from build123d import *
from build123d.topology import SkipClean

# Parameters (mm, degrees)
BOSS_EXTRUDE1_DEPTH     = 50
BOSS_EXTRUDE2_START     = 9
BOSS_EXTRUDE2_DEPTH     = 9
BOSS_EXTRUDE3_START     = 9
BOSS_EXTRUDE3_DEPTH     = 9
BOSS_EXTRUDE4_DEPTH     = 70
CUT_EXTRUDE2_DEPTH      = 165.74298164110058
CUT_EXTRUDE2_DEPTH_BACK = 165.74298164110058
SKETCH10_W              = 30.000000000000007
SKETCH10_H              = 30
SKETCH10_W_2            = 30.00000000000001
SKETCH10_H_2            = 29.999999999999996
BOSS_EXTRUDE7_DEPTH     = 90
BOSS_EXTRUDE8_DEPTH     = 235
SKETCH12_W              = 24.999999999999993
SKETCH12_H              = 40.90326072663956
SKETCH12_H_2            = 38.73852460954424
SKETCH12_W_2            = 25.000000000000007
SKETCH12_H_3            = 39.91957718910348
CUT_EXTRUDE3_DEPTH      = 235
SKETCH13_R              = 7.499999999999999
CUT_EXTRUDE4_DEPTH      = 235
FILLET1_R               = 10


with BuildPart() as part:
    # Sketch1 → Boss-Extrude1 (new body)
    with BuildSketch(Plane(origin=(0, 0, 0), x_dir=(0, 0, -1), z_dir=(1, 0, 0))):
        with BuildLine():
            Line((-130.5, 0), (130.5, 0))
            ThreePointArc((130.5, 0), (137.57106781186548, -2.9289321881345245), (140.5, -9.999999999999998))
            Line((140.5, -9.999999999999998), (140.5, -69.99999999999999))
            Line((140.5, -69.99999999999999), (122.5, -70))
            ThreePointArc((122.5, -70), (97.5, -45), (72.50000000000001, -70))
            Line((72.50000000000001, -70), (57.5, -70))
            ThreePointArc((57.5, -70), (32.5, -45), (7.5, -70))
            Line((7.5, -70), (-7.5, -70))
            ThreePointArc((-7.5, -70), (-32.5, -45), (-57.5, -70))
            Line((-57.5, -70), (-72.50000000000001, -70))
            ThreePointArc((-72.50000000000001, -70), (-97.5, -45), (-122.5, -70))
            Line((-122.5, -70), (-140.5, -69.99999999999999))
            Line((-140.5, -69.99999999999999), (-140.5, -9.999999999999998))
            ThreePointArc((-140.5, -9.999999999999998), (-137.57106781186548, -2.9289321881345245), (-130.5, 0))
        make_face()
    extrude(amount=BOSS_EXTRUDE1_DEPTH)

    # Sketch2 → Boss-Extrude2 (add)
    with BuildSketch(Plane.ZY.offset(BOSS_EXTRUDE2_START)):
        with BuildLine():
            Line((0, 0), (130.5, 0))
            ThreePointArc((130.5, 0), (137.57106781186548, -2.9289321881345236), (140.5, -9.999999999999998))
            Line((140.5, -9.999999999999998), (140.5, -69.99999999999999))
            Line((140.5, -69.99999999999999), (135.5, -69.99999999999999))
            Line((135.5, -69.99999999999999), (135.5, -15))
            ThreePointArc((135.5, -15), (132.57106781186548, -7.928932188134525), (125.5, -5.000000000000002))
            Line((125.5, -5.000000000000002), (0, -5.000000000000017))
            Line((0, -5.000000000000017), (0, 0))
        make_face()
    extrude(amount=-BOSS_EXTRUDE2_DEPTH)

    # Sketch3 → Boss-Extrude3 (add)
    with BuildSketch(Plane.ZY.offset(BOSS_EXTRUDE3_START)):
        with BuildLine():
            Line((0, 0), (0, -5.000000000000017))
            Line((0, -5.000000000000017), (-125.5, -5.000000000000032))
            ThreePointArc((-125.5, -5.000000000000032), (-132.57106781186548, -7.9289321881345565), (-135.5, -15.000000000000034))
            Line((-135.5, -15.000000000000034), (-135.5, -69.99999999999999))
            Line((-135.5, -69.99999999999999), (-140.5, -69.99999999999999))
            Line((-140.5, -69.99999999999999), (-140.5, -10.00000000000007))
            ThreePointArc((-140.5, -10.00000000000007), (-137.5710678118655, -2.9289321881345742), (-130.50000000000003, 5.2e-15))
            Line((-130.50000000000003, 5.2e-15), (0, 0))
        make_face()
    extrude(amount=-BOSS_EXTRUDE3_DEPTH)

    # Sketch6 → Boss-Extrude4 (add)
    with BuildSketch(Plane(origin=(0, 0, 0), x_dir=(1, 0, 0), z_dir=(0, 1, 0))):
        Polygon((50, -140.5), (50, 140.5), (43, 140.5), (43.000000000000036, -140.5), align=None)
    extrude(amount=-BOSS_EXTRUDE4_DEPTH)

    # Sketch9 → Cut-Extrude2 (cut, two sides: drawn at the far end of the back side and taken through both)
    with BuildSketch(Plane(origin=(0, 0, 0), x_dir=(1, 0, 0), z_dir=(0, 1, 0)).offset(-CUT_EXTRUDE2_DEPTH_BACK)):
        Polygon((40.000000000000675, 47.5), (40.00000000000068, 17.49999999999999), (10.000000000000675, 17.49999999999999), (10.000000000000671, 47.499999999999986), align=None)
        Polygon((39.99999999999999, 112.5), (9.999999999999995, 112.49999999999999), (9.999999999999998, 82.49999999999999), (40, 82.49999999999999), align=None)
        Polygon((40.00000000000135, -17.5), (40.00000000000136, -47.500000000000014), (10.000000000001352, -47.500000000000014), (10.000000000001348, -17.500000000000014), align=None)
        Polygon((40.000000000002025, -82.5), (40.00000000000203, -112.50000000000001), (10.00000000000203, -112.50000000000001), (10.000000000002027, -82.50000000000001), align=None)
    extrude(amount=CUT_EXTRUDE2_DEPTH + CUT_EXTRUDE2_DEPTH_BACK, mode=Mode.SUBTRACT)

    # Sketch10 → Boss-Extrude7 (add)
    # profile 1 of 4: a face of its own
    with BuildSketch(Plane(origin=(0, 0, 0), x_dir=(1, 0, 0), z_dir=(0, 1, 0))):
        Polygon((4.99999999999999, 117.5), (44.99999999999999, 117.5), (45, 77.49999999999999), (4.999999999999995, 77.49999999999999), align=None)
        with Locations((24.999999999999996, 97.49999999999999)):
            Rectangle(SKETCH10_W, SKETCH10_H, mode=Mode.SUBTRACT)
    # profile 2 of 4: a face of its own
    with BuildSketch(Plane(origin=(0, 0, 0), x_dir=(1, 0, 0), z_dir=(0, 1, 0))):
        Polygon((5.000000000000667, 52.49999999999999), (5.0000000000006715, 12.499999999999984), (45.000000000000675, 12.499999999999984), (45.00000000000067, 52.49999999999999), align=None)
        with Locations((25.000000000000675, 32.499999999999986)):
            Rectangle(SKETCH10_W_2, SKETCH10_H_2, mode=Mode.SUBTRACT)
    # profile 3 of 4: a face of its own
    with BuildSketch(Plane(origin=(0, 0, 0), x_dir=(1, 0, 0), z_dir=(0, 1, 0))):
        Polygon((5.000000000001345, -12.50000000000001), (5.000000000001349, -52.50000000000002), (45.00000000000135, -52.50000000000002), (45.00000000000134, -12.50000000000001), align=None)
        with Locations((25.000000000001354, -32.500000000000014)):
            Rectangle(SKETCH10_W, SKETCH10_H, mode=Mode.SUBTRACT)
    # profile 4 of 4: a face of its own
    with BuildSketch(Plane(origin=(0, 0, 0), x_dir=(1, 0, 0), z_dir=(0, 1, 0))):
        Polygon((5.0000000000020215, -77.50000000000001), (5.000000000002025, -117.50000000000001), (45.00000000000203, -117.50000000000001), (45.000000000002025, -77.50000000000001), align=None)
        with Locations((25.00000000000203, -97.50000000000001)):
            Rectangle(SKETCH10_W, SKETCH10_H, mode=Mode.SUBTRACT)
    extrude(amount=BOSS_EXTRUDE7_DEPTH)

    # Sketch11 → Boss-Extrude8 (add)
    with BuildSketch(Plane.XY.offset(117.50000000000001)):
        with BuildLine():
            Line((45.00000000000203, 59.449874371066194), (45.00000000000203, 56.93303437365923))
            ThreePointArc((45.00000000000203, 56.93303437365923), (53.50000000000204, 49.499999999999986), (45.00000000000203, 42.06696562634074))
            Line((45.00000000000203, 42.06696562634074), (45.00000000000203, 39.55012562893379))
            ThreePointArc((45.00000000000203, 39.5501256289338), (56.000000000002046, 49.5), (45.00000000000203, 59.4498743710662))
        make_face()
    extrude(amount=-BOSS_EXTRUDE8_DEPTH)

    # Sketch12 → Cut-Extrude3 (cut)
    with BuildSketch(Plane(origin=(0, 0, 0), x_dir=(0, 0, -1), z_dir=(1, 0, 0))):
        with Locations((-65.00000000000001, 54.273306822213314)):
            Rectangle(SKETCH12_W, SKETCH12_H)
        with Locations((-1.421e-14, 51.301254636370814)):
            Rectangle(SKETCH12_W, SKETCH12_H_2)
        with Locations((65, 47.16757060791335)):
            Rectangle(SKETCH12_W_2, SKETCH12_H_3)
    extrude(amount=CUT_EXTRUDE3_DEPTH, mode=Mode.SUBTRACT)

    # Sketch13 → Cut-Extrude4 (cut)
    with SkipClean():  # the faces are left unmerged after this step: merging them gives an invalid solid
        with BuildSketch(Plane.XY.offset(117.50000000000001)):
            with Locations((46.000000000002046, 49.499999999999986)):
                Circle(SKETCH13_R)
        extrude(amount=-CUT_EXTRUDE4_DEPTH, mode=Mode.SUBTRACT)

    # Fillet1
    fillet1_edges = [part.edges().sort_by_distance(p)[0] for p in [
        (46.500000000000014, 0, 140.5),
        (46.5, 0, -140.5),
    ]]
    fillet(fillet1_edges, radius=FILLET1_R)


solid = part.part
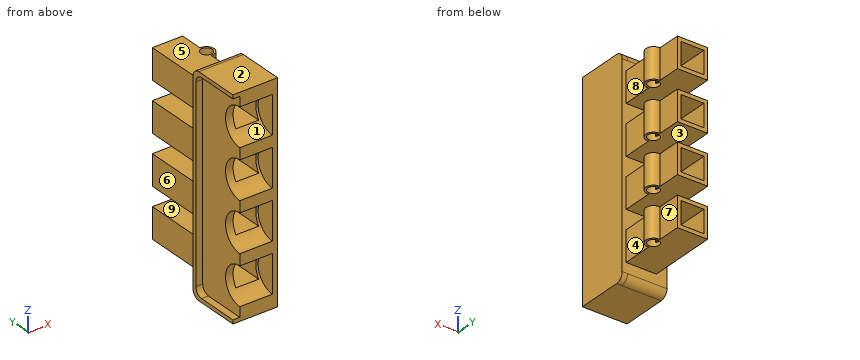
Input: part model. Units: mm. Frame: model coordinates. Face numbers are marked on the shaded views. A direction names the side the tool comes from. Round coordinates to 2 decimals unless told otherwise and drop trailing zeros. Loops run counter-clockwise (first coordinate to the right, second up) from the corner with the lowest first, then second, coordinate; pieces in that order, holes last. Notation, with made-up numbers: M 8,70.5 L 33,70.5 A24 ccw 33,88.5 Z; hole C -18,45.25 d2. An arc over 180 degrees is marked long. Answer as CSV lines item,"result". Start each with the question number.
(1) Reachability of the marked faces 5, 6, 7, 8 and 9 from +Z, -Z, +X, -X, +Y, -Y: full face, straight path, thin tool, end or side. Return the list, or none.
(2) Section C-C, the plane y = -41.5. Output: boundary loops of the cut face in (x, z).
(3) Section B-B, the plane z = -32.5. Output: boundary loops of the cut face in (x, y), plus the area to 3 significant figures.
(4) Section A-A, the plane y = 62.5. State how many separate pieces and enclosed holes the cut face has, plus the area to 3 significant figures.
(5) Draft query along Z for the marked faces 1, 2, 3 and 4. Return one class per face: released by +Z, released by -Z, zero draft, split by the parting line, or undercut.
(6) Line query: line 1 (Z direction, x = 35.5, y = -24); line 2 (Z direction, x = 41.5, y = 26); line 3 (Y direction, x = 46, z = -32). Output: solid intervals per line, ascending. Write a range as [from, to].
(7) First-contact query: pin 1 (8 mm diameter, centred on x = 23, y = 33, fed in from +Z); pin 2 (8 mm diameter, centred on y = 10, z = 102, fed in from +X); pin 3 (10 mm diameter, centred on x = 44.5, y = 54.5, fed in from -Z). Flat tips, straight axial feed; report the tip coordinate or a pass-through.
Values found:
1,face 5,"+Z, +X, -X, +Y"
1,face 6,"+Z, -Z, -X, +Y"
1,face 7,"+Z, -Z, +X, +Y"
1,face 8,"+Z, -Z, +X"
1,face 9,"+X, -X, +Y"
2,outline,"M -9,-140.5 L 50,-140.5 L 50,140.5 L -9,140.5 L -9,135.5 L 0,135.5 L 0,-135.5 L -9,-135.5 Z; hole M 10,-112.5 L 40,-112.5 L 40,-82.5 L 10,-82.5 Z; hole M 10,-47.5 L 40,-47.5 L 40,-17.5 L 10,-17.5 Z; hole M 10,17.5 L 40,17.5 L 40,47.5 L 10,47.5 Z; hole M 10,82.5 L 40,82.5 L 40,112.5 L 10,112.5 Z"
3,outline,"M -9,-5 L 0,-5 L 0,-45 L 10,-45 L 10,90 L 5,90 L 5,0 L -9,0 Z; M 40,-45 L 43,-45 L 43,-70 L 50,-70 L 50,0 L 45,0 L 45,39.55 A10 ccw long 45,59.45 L 45,90 L 40,90 L 40,54 A7.5 cw long 40,45 Z"
3,area,"2,030 mm²"
4,separate pieces,"4"
4,enclosed holes,"4"
4,area,"2,800 mm²"
5,face 1,"undercut"
5,face 2,"released by +Z"
5,face 3,"undercut"
5,face 4,"zero draft"
6,line 1,"z = [-140.5, -112.5], [-82.5, -47.5], [-17.5, 17.5], [47.5, 82.5], [112.5, 140.5]"
6,line 2,"z = [-117.5, -77.5], [-52.5, -12.5], [12.5, 52.5], [77.5, 117.5]"
6,line 3,"y = [-70, 0], [39.5, 42], [57, 59.5]"
7,pin 1,"stops at z = 117.5"
7,pin 2,"stops at x = 45"
7,pin 3,"stops at z = -117.5"
